```python
from build123d import *

# Parameters (mm, degrees)
BOSS_EXTRUDE1_DEPTH = 3
CUT_EXTRUDE3_DEPTH  = 535.143239216
SKETCH6_W           = 330
SKETCH6_H           = 70
CUT_EXTRUDE4_DEPTH  = 467.700117849
FILLET1_R           = 10


with BuildPart() as part:
    # Sketch3 → Boss-Extrude1 (new body)
    with BuildSketch(Plane(origin=(0, 0, 0), x_dir=(1, 0, 0), z_dir=(0, 1, 0))):
        with BuildLine():
            Line((-36.319194267, -89.236860887), (144.478790315, -23.431776084))
            ThreePointArc((144.478790315, -23.431776084), (165.000000077, -19.813332936), (185.52120983, -23.431776136))
            Line((185.52120983, -23.431776136), (366.319192052, -89.236860081))
            ThreePointArc((366.319192052, -89.236860081), (416.877444894, -67.142834059), (397.269838057, -15.569346002))
            Line((397.269838057, -15.569346002), (344.206351456, 9.829836443))
            ThreePointArc((344.206351456, 9.829836443), (333.847680817, 19.053826006), (330, 32.379717841))
            Line((330, 32.379717841), (330, 330))
            Line((330, 330), (0, 330))
            Line((0, 330), (0, 32.379717841))
            ThreePointArc((0, 32.379717841), (-3.847681031, 19.053825667), (-14.206352179, 9.829836096))
            Line((-14.206352179, 9.829836096), (-67.269835876, -15.569344958))
            ThreePointArc((-67.269835876, -15.569344958), (-86.877445819, -67.142831858), (-36.319194267, -89.236860887))
        make_face()
    extrude(amount=BOSS_EXTRUDE1_DEPTH)

    # Sketch5 → Cut-Extrude3 (cut, through all)
    with BuildSketch(Plane(origin=(0, 0, 0), x_dir=(1, 0, 0), z_dir=(0, 1, 0))):
        Polygon((330, -1291.92309226), (330, -91.649156055), (330, 58.350843945), (420, 58.350843945), (420, -91.649156055), (-90, -91.649156055), (-90, 58.350843945), (0, 58.350843945), (0, -91.649156055), (0, -1291.92309226), (0, -3692.47096467), (330, -3692.47096467), align=None)
    extrude(amount=CUT_EXTRUDE3_DEPTH, mode=Mode.SUBTRACT)


with BuildPart() as cut_extrude3_kept_piece:
    # of the separate pieces the step leaves, the one the design keeps (cut_extrude3_pieces_kept)
    add(part.part.solids().sort_by_distance((0, 0, -330))[0])

    # Sketch6 → Cut-Extrude4 (cut, through all)
    with BuildSketch(Plane(origin=(0, 3, 0), x_dir=(1, 0, 0), z_dir=(0, 1, 0))):
        with Locations((165, 295)):
            Rectangle(SKETCH6_W, SKETCH6_H)
    extrude(amount=-CUT_EXTRUDE4_DEPTH, mode=Mode.SUBTRACT)

    # Fillet1
    fillet1_edges = [cut_extrude3_kept_piece.edges().sort_by_distance(p)[0] for p in [
        (330, 1.5, 76.017755241),
        (0, 1.5, -260),
        (330, 1.5, -260),
        (0, 1.5, 76.017755241),
    ]]
    fillet(fillet1_edges, radius=FILLET1_R)


solid = cut_extrude3_kept_piece.part
```
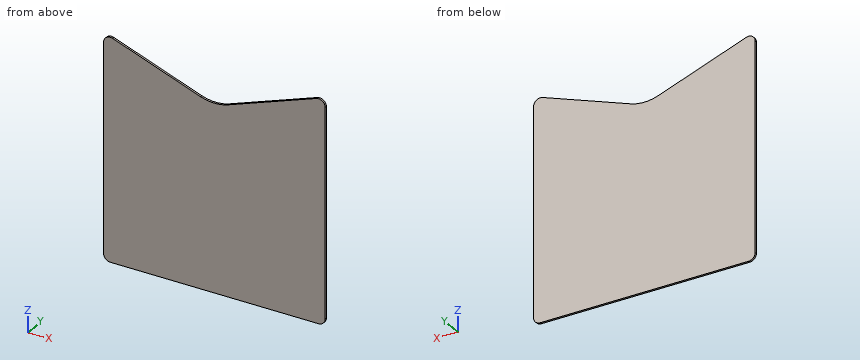
For this review, take the finished solid that the model builds, in its own axes (mm). Coordinates: 2 decimals unless noted, no trailing zeros. Write each loop counter-clockwise with the first axis right and the second up, starting at its lowest first coordinate (ties: lowest second). Pieces come first, ordered by that corner, then holes. Notation, with made-up numbers: (57.25, 6.5) - (82.25, 6.5) arc R19 cw to (82.25, 37.5) - close; hole circle Ø7 at (19, 9.25). An arc over 180 degrees is marked (long way). Answer in a Markdown table with one row per item. Add a question column.
Q1. For probe 1 along Z at (x, y) = (163.5, 1); probe 2 along Z at (x, y) = (316.5, 1.1), list the stretches that pass through material, from the lowest coordinate up.
Q2. For P1, Ø1, axis at x = 226.5, y = 0.5, coming from the +Z side, flat-tipped, find the tip position at first contact; note if it passes through.
Q3. We need section A-A, the plane y = 2.3. State the section outline as (x, z) points, and give its area (3 significant figures).
Q4. We need section B-B, the plane x = 49. State the section outline as (y, z) points, and give its area (3 significant figures).
Q5. We need section C-C, the plane x = 90. State the section outline as (y, z) points.
Answer list:
| question | item | result |
|---|---|---|
| 1 | probe 1 | z = -260 to 19.83 |
| 1 | probe 2 | z = -260 to 71.1 |
| 2 | P1 | stops at z = 38.53 |
| 3 | outline | (0, -250) arc R10 ccw to (10, -260) - (320, -260) arc R10 ccw to (330, -250) - (330, 61.74) arc R10 ccw to (316.58, 71.13) - (185.52, 23.43) arc R60 cw to (144.48, 23.43) - (13.42, 71.13) arc R10 ccw to (0, 61.74) - close |
| 3 | area | 101,000 mm2 |
| 4 | outline | (0, -260) - (3, -260) - (3, 58.18) - (0, 58.18) - close |
| 4 | area | 955 mm2 |
| 5 | outline | (0, -260) - (3, -260) - (3, 43.26) - (0, 43.26) - close |
